from build123d import *

# Parameters (mm, degrees)
SKETCH005_W     = 71.8
SKETCH005_H     = 45
SKETCH005_W_2   = 15.24
SKETCH005_H_2   = 2.54
SKETCH005_W_3   = 5.08
SKETCH005_H_3   = 38.1
PAD003_DEPTH    = 2
SKETCH006_W     = 71.8
SKETCH006_H     = 1.4
PAD004_DEPTH    = 3.3
SKETCH007_W     = 7
SKETCH007_H     = 22.5
PAD005_DEPTH    = 2.3
SKETCH010_W     = 5
SKETCH010_H     = 2.3
PAD006_DEPTH    = 0.4
SKETCH011_W     = 5
SKETCH011_H     = 2.3
PAD007_DEPTH    = 0.4
CHAMFER_SIZE    = 0.399
CHAMFER001_SIZE = 2


with BuildPart() as part:
    # Sketch005 → Pad003 (new body)
    with BuildSketch(Plane.XY.offset(4.3)):
        with Locations((-31.9, 0)):
            Rectangle(SKETCH005_W, SKETCH005_H)
        with Locations((-55, 18)):
            Rectangle(SKETCH005_W_2, SKETCH005_H_2, mode=Mode.SUBTRACT)
        with Locations((-55.5, -18)):
            Rectangle(SKETCH005_W_2, SKETCH005_H_2, mode=Mode.SUBTRACT)
        with Locations((-37, -18)):
            Rectangle(SKETCH005_W_2, SKETCH005_H_2, mode=Mode.SUBTRACT)
        with Locations((-12, 0)):
            Rectangle(SKETCH005_W_3, SKETCH005_H_3, mode=Mode.SUBTRACT)
    extrude(amount=PAD003_DEPTH)

    # Sketch006 (on Face21 of Pad003) → Pad004 (join)
    with BuildSketch(Plane(origin=(0, 0, 4.3), x_dir=(1, 0, 0), z_dir=(0, 0, -1))):
        with Locations((-31.9, 21.8)):
            Rectangle(SKETCH006_W, SKETCH006_H)
        with Locations((-31.9, -21.8)):
            Rectangle(SKETCH006_W, SKETCH006_H)
    extrude(amount=PAD004_DEPTH)

    # Sketch007 (on Face5 of Pad004) → Pad005 (join)
    with BuildSketch(Plane(origin=(0, 0, 4.3), x_dir=(1, 0, 0), z_dir=(0, 0, -1))):
        with Locations((0.5, 0)):
            Rectangle(SKETCH007_W, SKETCH007_H)
    extrude(amount=PAD005_DEPTH)

    # Sketch010 (on Face11 of Pad005) → Pad006 (join)
    with BuildSketch(Plane.XZ.offset(-21.1)):
        with Locations((0, 2.65)):
            Rectangle(SKETCH010_W, SKETCH010_H)
        with Locations((-63.8, 2.65)):
            Rectangle(SKETCH010_W, SKETCH010_H)
    extrude(amount=PAD006_DEPTH)

    # Sketch011 (on Face16 of Pad006) → Pad007 (join)
    with BuildSketch(Plane(origin=(0, -21.1, 0), x_dir=(-1, 0, 0), z_dir=(0, 1, 0))):
        with Locations((0, 2.65)):
            Rectangle(SKETCH011_W, SKETCH011_H)
        with Locations((63.8, 2.65)):
            Rectangle(SKETCH011_W, SKETCH011_H)
    extrude(amount=PAD007_DEPTH)

    # Chamfer
    chamfer_edges = [part.edges().sort_by_distance(p)[0] for p in [
        (-63.8, -20.7, 1.5),
        (0, -20.7, 1.5),
        (-63.8, 20.7, 1.5),
        (0, 20.7, 1.5),
    ]]
    chamfer(chamfer_edges, length=CHAMFER_SIZE)

    # Chamfer001
    chamfer001_edges = [part.edges().sort_by_distance(p)[0] for p in [
        (-31.9, 22.5, 6.3),
        (-31.9, -22.5, 6.3),
    ]]
    chamfer(chamfer001_edges, length=CHAMFER001_SIZE)


solid = part.part
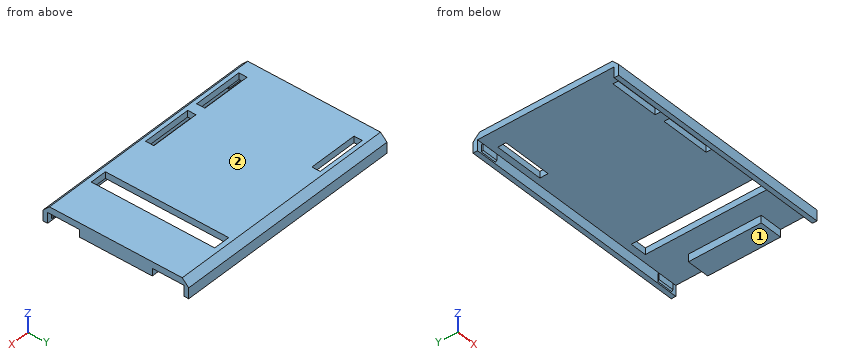
Geometry: final body of the model. Coordinates: model frame, mm. Face numbers are marked on the shaded views. Give positions to 0.01 mm unless a question says otherwise; leave off trailing zeros. Loops run counter-clockwise (first coordinate to the right, second up) from the corner with the lowest first, then second, coordinate; pieces in that order, holes last. Notation, with made-up numbers: (62, -17) - (92, -17) arc R23 ccw to (92, 2) - close; hole circle Ø5 at (-37.75, 39). An arc over 180 degrees is marked (long way). Answer as CSV lines item,"result". Start each with the question number.
1. Section D-D, the plane x = -49. Return loops of the section in (y, z).
2. Section B-B, the plane x = -10.5. Return loops of the section in (y, z), plus the area to 3 significant figures.
3. Ray query, L1, parallel to X at y = -17, z = 5.4; L2, parallel to X at y = 16.5, z = 4.7; L3, parallel to Y at x = -22, z = 2.95. Return the intervals inside material, ascending.
4. Pin query (flat end, axial travel): P1, Ø2, axis at x = -52, z = 5.5, coming from the -Y side; P2, Ø1.5, axis at x = -4.5, y = -15, coming from the -Z side; P3, Ø1.6, axis at x = -34.5, z = 5, coming from the -Y side; P4, Ø0.6, axis at x = -59, z = 5.5, coming from the +Y side. Return the tip coordinate at first contact, or that it passes through.
5. Section A-A, the plane y = -14.5. Return loops of the section in (x, z), plus the area to 3 significant figures.
6. Draft query along Y for the marked faces 1 and 2. Return one class per face: released by +Y, released by -Y, zero draft, split by the parting line, or undercut.
7. Section C-C, the plane z = 5.45. Return loops of the section in (x, y), plus the area to 3 significant figures.
Answers:
1,outline,"(-22.5, 1) - (-21.1, 1) - (-21.1, 4.3) - (-19.27, 4.3) - (-19.27, 6.3) - (-20.5, 6.3) - (-22.5, 4.3) - close; (-16.73, 4.3) - (16.73, 4.3) - (16.73, 6.3) - (-16.73, 6.3) - close; (19.27, 4.3) - (21.1, 4.3) - (21.1, 1) - (22.5, 1) - (22.5, 4.3) - (20.5, 6.3) - (19.27, 6.3) - close"
2,outline,"(-22.5, 1) - (-21.1, 1) - (-21.1, 4.3) - (-19.05, 4.3) - (-19.05, 6.3) - (-20.5, 6.3) - (-22.5, 4.3) - close; (19.05, 4.3) - (21.1, 4.3) - (21.1, 1) - (22.5, 1) - (22.5, 4.3) - (20.5, 6.3) - (19.05, 6.3) - close"
2,area,"19.0 mm2"
3,L1,"x = -67.8 to -63.12, -47.88 to -44.62, -29.38 to -14.54, -9.46 to 4"
3,L2,"x = -67.8 to -14.54, -9.46 to 4"
3,L3,"y = -22.5 to -21.1, 21.1 to 22.5"
4,P1,"stops at y = -22.3"
4,P2,"stops at z = 4.3"
4,P3,"stops at y = -22.5"
4,P4,"stops at y = 21.6"
5,outline,"(-67.8, 4.3) - (-14.54, 4.3) - (-14.54, 6.3) - (-67.8, 6.3) - close; (-9.46, 4.3) - (4, 4.3) - (4, 6.3) - (-9.46, 6.3) - close"
5,area,"133 mm2"
6,face 1,"undercut"
6,face 2,"zero draft"
7,outline,"(-67.8, -21.35) - (4, -21.35) - (4, 21.35) - (-67.8, 21.35) - close; hole (-63.12, -19.27) - (-47.88, -19.27) - (-47.88, -16.73) - (-63.12, -16.73) - close; hole (-62.62, 16.73) - (-47.38, 16.73) - (-47.38, 19.27) - (-62.62, 19.27) - close; hole (-44.62, -19.27) - (-29.38, -19.27) - (-29.38, -16.73) - (-44.62, -16.73) - close; hole (-14.54, -19.05) - (-9.46, -19.05) - (-9.46, 19.05) - (-14.54, 19.05) - close"
7,area,"2,760 mm2"
